```python
from build123d import *

# Parameters (mm, degrees)
F1_DEPTH = 0.6096
F2_W     = 3.4798
F2_H     = 1.9431
F3_DEPTH = 25.4
F5_SIZE2 = 1.5875
F5_SIZE  = 0.3042678278


with BuildPart() as f1:
    # F0 (on Front) → F1 (new body)
    with BuildSketch(Plane.XZ):
        Polygon((0, 19.05), (0, 0), (31.75, 0), (20.7514773719, 19.05), align=None)
    extrude(amount=F1_DEPTH)

    # F2 (on Front) → F3 (cut)
    with BuildSketch(Plane.XZ):
        with BuildLine():
            ThreePointArc((1.4224, 17.1069), (3.1623, 15.367), (4.9022, 17.1069))
            Line((4.9022, 17.1069), (1.4224, 17.1069))
        make_face()
        with Locations((3.1623, 18.07845)):
            Rectangle(F2_W, F2_H)
    extrude(amount=F3_DEPTH, mode=Mode.SUBTRACT)

    # F4: F1 across plane


with BuildPart() as f1_1:
    add(f1.part)
    add(f1.part.mirror(Plane.YZ))

    # F5
    f5_edges = [f1_1.edges().sort_by_distance(p)[0] for p in [
        (0, 0, 0),
        (0, -0.6096, 0),
    ]]
    f5_side = f1_1.faces().sort_by_distance((0, -0.3048, 0))[0]
    chamfer(f5_edges, length=F5_SIZE, length2=F5_SIZE2, reference=f5_side)


solid = f1_1.part
```
Part model, mm, in its own coordinate system. Coordinates: 2 decimals unless noted, no trailing zeros. Write each loop counter-clockwise with the first axis right and the second up, starting at its lowest first coordinate (ties: lowest second). Pieces come first, ordered by that corner, then holes.
Item 1: Mould opens along X. For faces 1 (the face through (-3.124, -0.301, 15.367)), 2 (the face through (-26.33, -0.3, 9.39)), 3 (the face through (-0.44, -0.46, 0.8)) say: released by +X, released by -X, zero draft, split by the parting line, or undercut.
Item 2: Probe line 1 (X direction, y = -0.15, z = 17.75); line 2 (X direction, y = -0.45, z = 18.25); line 3 (X direction, y = -0.35, z = 14.75). List the from-to ranges inside material, lowest first.
Item 3: Slice it at B-B (y = -0.2). Write the cut outline in (x, z), and give its area (3 significant figures).
Item 4: Slice it at C-C (z = 5). Write the cut outline in (x, y), and give its area (3 significant figures).
Results found:
1. face 1: undercut
1. face 2: released by -X
1. face 3: zero draft
2. line 1: x = -21.5 to -4.9, -1.42 to 1.42, 4.9 to 21.5
2. line 2: x = -21.21 to -4.9, -1.42 to 1.42, 4.9 to 21.21
2. line 3: x = -23.23 to 23.23
3. outline: (-31.44, 0.54) - (31.44, 0.54) - (20.75, 19.05) - (4.9, 19.05) - (4.9, 17.11) arc R1.74 cw to (1.42, 17.11) - (1.42, 19.05) - (-1.42, 19.05) - (-1.42, 17.11) arc R1.74 cw to (-4.9, 17.11) - (-4.9, 19.05) - (-20.75, 19.05) - close
3. area: 943 mm2
4. outline: (-28.86, -0.61) - (28.86, -0.61) - (28.86, 0) - (-28.86, 0) - close
4. area: 35.2 mm2
